```python
from build123d import *

# Parameters (mm, degrees)
F1_DEPTH = 457.2
F2_W     = 50.8
F2_H     = 50.8
F3_DEPTH = 25.4


with BuildPart() as f1:
    # F0 (on Top) → F1 (new body)
    with BuildSketch(Plane.XY):
        Polygon((-82.997608, -24.226959), (-82.997608, -49.626959), (-32.197608, -49.626959), (-32.197608, 1.173041), (-57.597608, 1.173041), (-57.597608, -24.226959), align=None)
    extrude(amount=F1_DEPTH)

    # F2 (on face) → F3 (cut)
    with BuildSketch(Plane.YZ.offset(-32.197608)):
        with Locations((-24.226959, 431.8)):
            Rectangle(F2_W, F2_H)
        with Locations((-24.226959, 25.4)):
            Rectangle(F2_W, F2_H)
    extrude(amount=-F3_DEPTH, mode=Mode.SUBTRACT)


solid = f1.part
```
For this review, take the finished solid that the model builds, in its own axes (mm). A direction names the side the tool comes from. Coordinates: 2 decimals unless noted, no trailing zeros. Write each loop counter-clockwise with the first axis right and the second up, starting at its lowest first coordinate (ties: lowest second). Pieces come first, ordered by that corner, then holes. Notation, with made-up numbers: (-6, 34) -> (14, 34) arc R22 cw to (14, 55) -> close; hole circle Ø2 at (-16.75, 57.25). An arc over 180 degrees is marked (long way). Put each result on its own line as item: value.
Q1. Take a section at D-D, the plane z = 38.5. State the section outline as (x, y) points.
From the geometry:
outline: (-83, -49.63) -> (-57.6, -49.63) -> (-57.6, -24.23) -> (-83, -24.23) -> close
Q2. Clearance check with flat-ended pins moving along their axes: pin 1 Ø7.5 at (x, y) = (-44.5, -18.5) entering from +Z; pin 2 Ø20.5 at (x, y) = (-41, -28.5) entering from -Z; pin 3 Ø20.5 at (y, z) = (-42, 34.5) entering from +X. State where each tip first meets the part, or that it passes through.
From the geometry:
pin 1: stops at z = 406.4
pin 2: stops at z = 50.8
pin 3: stops at x = -57.6
Q3. Take a section at B-B, the plane y = -33.5. State the section outline as (x, z) points, then the cut area to 3 significant figures.
From the geometry:
outline: (-83, 0) -> (-57.6, 0) -> (-57.6, 50.8) -> (-32.2, 50.8) -> (-32.2, 406.4) -> (-57.6, 406.4) -> (-57.6, 457.2) -> (-83, 457.2) -> close
area: 20,600 mm2
Q4. Wall thickness on L1, parallel to Y at x = -78.5, z = 190.5; L2, parallel to X at y = -10, z = 197.5; L3, parallel to Z at x = -54, y = -30.5: over which ranges is each line inside the solid? List them lowest first.
From the geometry:
L1: y = -49.63 to -24.23
L2: x = -57.6 to -32.2
L3: z = 50.8 to 406.4
Q5. Tool access review of faces 1 (the flat face through (-57.598, -37, 26)), 2 (the flat face through (-45, -25, 406.4)), 3 (the flat face through (-57.598, -11, 226)): name each direction out of +Z, -Z, +X, -X, +Y, -Y from which nothing blocks a thin tool from reaching the whole face with its end or side.
From the geometry:
face 1: -Z, +X, +Y, -Y
face 2: +Z, +X, +Y, -Y
face 3: +Z, -Z, -X, +Y
Q6. Take a section at C-C, the plane x = -68. State the section outline as (y, z) points.
From the geometry:
outline: (-49.63, 0) -> (-24.23, 0) -> (-24.23, 457.2) -> (-49.63, 457.2) -> close
Q7. Take a section at A-A, the plane z = 267. State the section outline as (x, y) points.
From the geometry:
outline: (-83, -49.63) -> (-32.2, -49.63) -> (-32.2, 1.17) -> (-57.6, 1.17) -> (-57.6, -24.23) -> (-83, -24.23) -> close
